Could you check a few things on this model? Use its own coordinates, in mm. Face numbers are marked on the shaded views. A direction names the side the tool comes from. Coordinates: 2 decimals unless noted, no trailing zeros. Write each loop counter-clockwise with the first axis right and the second up, starting at its lowest first coordinate (ties: lowest second). Pieces come first, ordered by that corner, then holes. Notation, with made-up numbers: (12.25, 69) - (35.25, 69) arc R14 ccw to (35.25, 84) - close; hole circle Ø5 at (55.25, -5.75). An arc over 180 degrees is marked (long way). Answer as a JSON object with one key per item and string values. Group by question number.
1) On a 3-axis mill with a long thin cutter (end or side, diameter ignored), from which of +Z, -Z, +X, -X, +Y, -Y can I reach the whole of each face in a straight line? I mean the marked faces 1 and 2. Say none if no direction works.
2) Will these pins go through, and if not, where does the flat tip stop? pin 1 Ø4 at (x, y) = (62, -171) entering from +Z; pin 2 Ø23 at (x, y) = (60.1, -260) entering from +Z; pin 3 Ø9.5 at (y, z) = (-12.92, 234.97) entering from +X (3 decimals); pin 4 Ø6 at (x, z) = (47, 204) entering from -Y.
3) If we section it at B-B (z = 128): Write out the boundary of the cut face in (x, y).
4) Please list where these lines run through material, in increasing order: line 1 along Y through (x, z) = (57, 28); line 2 along Y through (x, z) = (56, 139.5); line 3 along Z through (x, y) = (-6, -144).
5) If we section it at C-C (x = 58): Write out the boundary of the cut face in (y, z), plus the area to 3 significant figures.
6) If we section it at A-A (y = -260): Write out the boundary of the cut face in (x, z), plus the area to 3 significant figures.
7) If we section it at D-D (y = -77): Write out the boundary of the cut face in (x, z), plus the area to 3 significant figures.
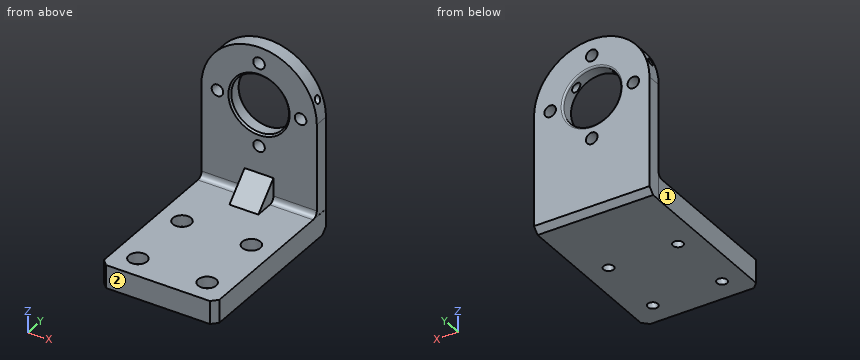
```python
from build123d import *

# Parameters (mm, degrees)
F0_R           = 10
F1_DEPTH       = 25
F2_D           = 20
F3_W           = 199.7033953667
F3_H           = 40
F4_DEPTH       = 300
F6_DEPTH       = 25
F8_D           = 17.5
F8_CBORE_D     = 31.5
F8_CBORE_DEPTH = 20
F9_SIZE        = 10
F10_SIZE       = 3
F11_R          = 3
F12_R          = 10
F14_D          = 12.1
F15_SIZE       = 10


with BuildPart() as f1:
    # F0 (on Front) → F1 (new body)
    with BuildSketch(Plane.XZ):
        with BuildLine():
            Line((-100, 200), (-100, 0))
            Line((-100, 0), (100, 0))
            Line((100, 0), (100, 200))
            Line((100, 200), (82, 200))
            ThreePointArc((82, 200), (72, 190), (62, 200))
            Line((62, 200), (50, 200))
            ThreePointArc((50, 200), (0, 150), (-50, 200))
            Line((-50, 200), (-62, 200))
            ThreePointArc((-62, 200), (-72, 190), (-82, 200))
            Line((-82, 200), (-100, 200))
        make_face()
        with Locations((0, 128)):
            Circle(F0_R, mode=Mode.SUBTRACT)
        with BuildLine():
            ThreePointArc((100, 200), (0, 300), (-100, 200))
            Line((-100, 200), (-82, 200))
            ThreePointArc((-82, 200), (-72, 210), (-62, 200))
            Line((-62, 200), (-50, 200))
            ThreePointArc((-50, 200), (0, 250), (50, 200))
            Line((50, 200), (62, 200))
            ThreePointArc((62, 200), (72, 210), (82, 200))
            Line((82, 200), (100, 200))
        make_face()
        with Locations((0, 272)):
            Circle(F0_R, mode=Mode.SUBTRACT)
        with BuildLine():
            ThreePointArc((62, 200), (72, 190), (82, 200))
            Line((82, 200), (62, 200))
        make_face()
        with BuildLine():
            Line((62, 200), (82, 200))
            ThreePointArc((82, 200), (72, 210), (62, 200))
        make_face()
        with BuildLine():
            ThreePointArc((-62, 200), (-72, 210), (-82, 200))
            Line((-82, 200), (-62, 200))
        make_face()
        with BuildLine():
            Line((-62, 200), (-82, 200))
            ThreePointArc((-82, 200), (-72, 190), (-62, 200))
        make_face()
        with Locations((0, 272)):
            Circle(F0_R)
        with Locations((0, 128)):
            Circle(F0_R)
    extrude(amount=F1_DEPTH)

    # F2 (through all)
    with Locations(Plane(origin=(0, 0, 0), x_dir=(1, 0, 0), z_dir=(0, 1, 0))):
        with Locations((0, -272), (72, -200), (0, -128), (-72, -200)):
            Hole(F2_D / 2)

    # F3 (on Front) → F4 (join)
    with BuildSketch(Plane.XZ):
        with Locations((0.2531558275, 20)):
            Rectangle(F3_W, F3_H)
    extrude(amount=F4_DEPTH)

    # F5 (on Right) → F6 (join, symmetric)
    with BuildSketch(Plane.YZ):
        Polygon((-66.1523267627, 40), (-25, 40), (-25, 81.1523267627), align=None)
    extrude(amount=F6_DEPTH, both=True)

    # F8 (through all)
    with Locations(Plane.XY.offset(40)):
        with Locations((-59.6462091353, -140.7010122926), (60.1048535109, -140), (60.1048535109, -260), (-59.8951464891, -260)):
            CounterBoreHole(F8_D / 2, F8_CBORE_D / 2, F8_CBORE_DEPTH)

    # F9
    f9_edges = [f1.edges().sort_by_distance(p)[0] for p in [
        (-99.598542, -300, 20),
        (100.104854, -300, 20),
    ]]
    chamfer(f9_edges, length=F9_SIZE)

    # F10
    f10_edges = [f1.edges().sort_by_distance(p)[0] for p in [
        (50, -25, 200),
    ]]
    chamfer(f10_edges, length=F10_SIZE)

    # F11
    f11_edges = [f1.edges().sort_by_distance(p)[0] for p in [
        (50, 0, 200),
    ]]
    fillet(f11_edges, radius=F11_R)

    # F12
    f12_edges = [f1.edges().sort_by_distance(p)[0] for p in [
        (-62.299271, -25, 40),
        (62.5, -25, 40),
    ]]
    fillet(f12_edges, radius=F12_R)

    # F14 (through all)
    with Locations(Plane(origin=(-100, 0, 0), x_dir=(0, -1, 0), z_dir=(-1, 0, 0))):
        with Locations((12.9178790376, 234.974578023)):
            Hole(F14_D / 2)

    # F15
    f15_edges = [f1.edges().sort_by_distance(p)[0] for p in [
        (0.052427, 0, 0),
    ]]
    chamfer(f15_edges, length=F15_SIZE)


solid = f1.part
```
Here are the results:
{
 "1": {"face 1": "+Z, -Z, -X, -Y", "face 2": "+Z, -Z, +X, -X, -Y"},
 "2": {"pin 1": "stops at z = 40", "pin 2": "stops at z = 20", "pin 3": "passes through", "pin 4": "stops at y = -22.17"},
 "3": {"outline": "(-100, -25) - (-10, -25) - (-10, 0) - (-100, 0) - close; (10, -25) - (100, -25) - (100, 0) - (10, 0) - close"},
 "4": {"line 1": "y = -300 to -275.44, -244.56 to -155.44, -124.56 to 0", "line 2": "y = -25 to 0", "line 3": "z = 0 to 40"},
 "5": {"outline": "(-300, 0) - (-268.49, 0) - (-268.49, 20) - (-275.61, 20) - (-275.61, 40) - (-300, 40) - close; (-251.51, 0) - (-148.49, 0) - (-148.49, 20) - (-155.61, 20) - (-155.61, 40) - (-244.39, 40) - (-244.39, 20) - (-251.51, 20) - close; (-131.51, 0) - (-10, 0) - (0, 10) - (0, 281.46) - (-25, 281.46) - (-25, 50) arc R10 cw to (-35, 40) - (-124.39, 40) - (-124.39, 20) - (-131.51, 20) - close; hole circle Ø12.1 at (-12.92, 234.97)", "area": "16,000 mm²"},
 "6": {"outline": "(-99.6, 0) - (-68.65, 0) - (-68.65, 20) - (-75.65, 20) - (-75.65, 40) - (-99.6, 40) - close; (-51.15, 0) - (51.35, 0) - (51.35, 20) - (44.35, 20) - (44.35, 40) - (-44.15, 40) - (-44.15, 20) - (-51.15, 20) - close; (68.85, 0) - (100.1, 0) - (100.1, 40) - (75.85, 40) - (75.85, 20) - (68.85, 20) - close", "area": "6,030 mm²"},
 "7": {"outline": "(-99.6, 0) - (100.1, 0) - (100.1, 40) - (-99.6, 40) - close", "area": "7,990 mm²"}
}
